from build123d import *

# Parameters (mm, degrees)
SKETCH2_R          = 26.5
CUT_EXTRUDE1_DEPTH = 2
CHAMFER1_SIZE      = 2
SKETCH3_R          = 16
CUT_EXTRUDE2_DEPTH = 83.076184122
CHAMFER3_SIZE      = 1


with BuildPart() as part:
    # Sketch1 → Revolve1 (revolve)
    with BuildSketch(Plane(origin=(0, 0, 0), x_dir=(1, 0, 0), z_dir=(0, 1, 0))):
        Polygon((0, 0), (70, 0), (70, -25.5), (35, -25.5), (35, -32.5), (28, -32.5), (28, -25), (7, -25), (7, -32.5), (0, -32.5), align=None)
    revolve(axis=Axis((0, 0, 0), (1, 0, 0)))

    # Sketch2 → Cut-Extrude1 (cut)
    with BuildSketch(Plane.ZY):
        Circle(SKETCH2_R)
    extrude(amount=-CUT_EXTRUDE1_DEPTH, mode=Mode.SUBTRACT)

    # Chamfer1
    chamfer1_edges = [part.edges().sort_by_distance(p)[0] for p in [
        (2, 0, -26.5),
    ]]
    chamfer(chamfer1_edges, length=CHAMFER1_SIZE - 0.0001)  # a hair under: the kernel refuses the full size

    # Sketch3 → Cut-Extrude2 (cut, through all)
    with BuildSketch(Plane.ZY.offset(-2)):
        Circle(SKETCH3_R)
    extrude(amount=-CUT_EXTRUDE2_DEPTH, mode=Mode.SUBTRACT)

    # Chamfer3
    chamfer3_edges = [part.edges().sort_by_distance(p)[0] for p in [
        (70, 0, -25.5),
    ]]
    chamfer(chamfer3_edges, length=CHAMFER3_SIZE)


solid = part.part
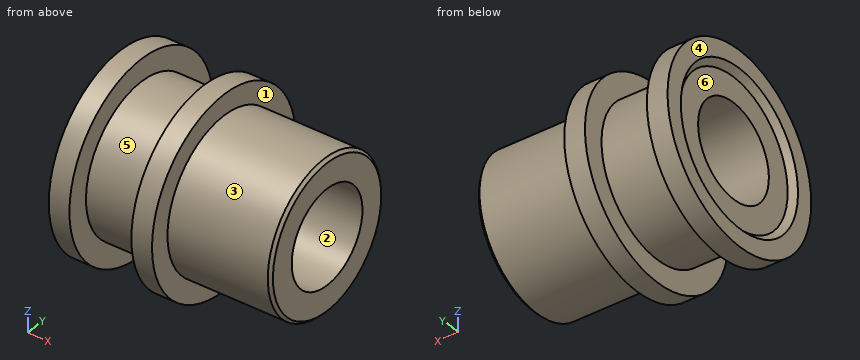
The listing builds one solid part. Answer for the finished solid, in the listing's coordinates (mm). Face numbers are marked on the shaded views. A direction names the side the tool comes from. Round coordinates to 2 decimals unless told otherwise and drop trailing zeros. Write each loop counter-clockwise with the first axis right and the second up, starting at its lowest first coordinate (ties: lowest second). Pieces come first, ordered by that corner, then holes. Notation, with made-up numbers: M -17.75,-15 L 17.25,-15 A20 cw 17.25,12 Z; hole C 73.25,-17 d1. An arc over 180 degrees is marked long. Write each question's results on one line, items separated by ' | '. Start each with the question number.
Item 1: For the marked faces 4, 5 and 6, determine the directions among +Z, -Z, +X, -X, +Y, -Y from which every point of the face is accessible in a straight line to the end or side of a thin tool.
Item 2: A cutting plane is placed at C-C on x = 33. Write down the section's boundary in (y, z), and give its area (3 significant figures).
Item 3: For a pull along Z with two mould halves and no side action, classify the marked faces 1, 2 and 3 as pulls with the +Z half, pulls with the -Z half, needs draft (parallel to the pull), parting line crosses it, or undercut.
Item 4: Straight lines are drawn through the part: L1, parallel to X at y = -16.5, z = -26.5; L2, parallel to Y at x = 17, z = 0; L3, parallel to X at y = -18, z = 5.5. For each, find the intervals that lie inside material, in ascending order. Write a range as [from, to].
Item 5: Flat-ended cylindrical pins translate along their axes: pin 1 Ø2 at (x, y) = (25, 18.5) entering from +Z; pin 2 Ø6 at (x, y) = (53, -18.5) entering from -Z; pin 3 Ø4 at (x, y) = (44.5, 4) entering from -Z. Find the tip coordinate at first contact, or state that the pin passes through.
Item 6: A cutting plane is placed at D-D on x = 46.5. Write down the section's boundary in (y, z).
Check sheet entries:
1) face 4: +Z, -Z, -X, +Y, -Y | face 5: none | face 6: -X
2) outline: C 0,0 d65; hole C 0,0 d32 | area: 2,510 mm²
3) face 1: needs draft | face 2: undercut | face 3: parting line crosses it
4) L1: [0, 7], [28, 35] | L2: [-25, -16], [16, 25] | L3: [2, 70]
5) pin 1: z = 17.85 | pin 2: z = -20.25 | pin 3: z = -25.42
6) outline: C 0,0 d51; hole C 0,0 d32
